Source: CAD feature listing. Evaluate the final solid. Frame: model axes, mm. A direction names the side the tool comes from. Give positions to 0.01 mm unless a question says otherwise; leave off trailing zeros. Loops run counter-clockwise (first coordinate to the right, second up) from the corner with the lowest first, then second, coordinate; pieces in that order, holes last.
```python
from build123d import *

# Parameters (mm, degrees)
F0_W     = 6.35
F0_H     = 34.29
F1_DEPTH = 9.525
F3_DEPTH = 6.351


with BuildPart() as f1:
    # F0 (on Top) → F1 (new body)
    with BuildSketch(Plane.XY):
        Rectangle(F0_W, F0_H)
    extrude(amount=F1_DEPTH)

    # F2 (on face) → F3 (cut, through all)
    with BuildSketch(Plane(origin=(-3.175, 0, 0), x_dir=(0, -1, 0), z_dir=(-1, 0, 0))):
        Polygon((-17.145, 9.525), (-17.145, 6.35), (-10.795, 6.35), (-13.97, 9.525), align=None)
        Polygon((17.145, 9.525), (13.97, 9.525), (10.795, 6.35), (17.145, 6.35), align=None)
    extrude(amount=-F3_DEPTH, mode=Mode.SUBTRACT)


solid = f1.part
```
(1) Section A-A, the plane y = 12. Return the cut outline in (x, z) (3 decimals), then the cut area to 3 significant figures.
A:
outline: (-3.175, 0) - (3.175, 0) - (3.175, 6.35) - (-3.175, 6.35) - close; (-3.175, 7.555) - (3.175, 7.555) - (3.175, 9.525) - (-3.175, 9.525) - close
area: 52.8 mm2
(2) Section C-C, the plane y = -13. Return the cut outline in (x, z) (3 decimals), then the cut area to 3 significant figures.
A:
outline: (-3.175, 0) - (3.175, 0) - (3.175, 6.35) - (-3.175, 6.35) - close; (-3.175, 8.555) - (3.175, 8.555) - (3.175, 9.525) - (-3.175, 9.525) - close
area: 46.5 mm2
(3) Section B-B, the plane x = -2. Return the cut outline in (y, z) (3 decimals).
A:
outline: (-17.145, 0) - (17.145, 0) - (17.145, 6.35) - (10.795, 6.35) - (13.97, 9.525) - (-13.97, 9.525) - (-10.795, 6.35) - (-17.145, 6.35) - close
(4) Reachability of faces 5 (the flat face through (0, -14, 6.35)), 6 (the flat face through (-0.044, 12.36, 7.915)), 7 (the flat face through (0, 0, 9.525)) from +Z, -Z, +X, -X, +Y, -Y: full face, straight path, thin tool, end or side. Return the list, or none.
A:
face 5: +X, -X, -Y
face 6: +X, -X, +Y
face 7: +Z, +X, -X, +Y, -Y
(5) Section D-D, the plane z = 8.5. Return the cut outline in (x, y) (3 decimals), then the cut area to 3 significant figures.
A:
outline: (-3.175, -12.945) - (3.175, -12.945) - (3.175, 12.945) - (-3.175, 12.945) - close
area: 164 mm2
(6) First-contact query: pin 1 (1.9 mm diameter, centred on x = 1.5, y = 15, fed in from +Z). Flat tip, straight axial feed; report the tip coordinate or a pass-through.
A:
pin 1: stops at z = 6.35
(7) Ray query, line 1 along Z through (x, y) = (1.5, -12.5) (3 decimals); line 2 along Z through (x, y) = (-0.5, -11.5) (3 decimals); line 3 along Z through (x, y) = (-2.5, 15). Return the intervals inside material, ascending.
A:
line 1: z = 0 to 6.35, 8.055 to 9.525
line 2: z = 0 to 6.35, 7.055 to 9.525
line 3: z = 0 to 6.35
(8) Mould query, pull axis Z, two halves, no side actions, for faces 1 (the flat face through (-0.044, -12.405, 7.96)), 2 (the flat face through (0, 14, 6.35)), 3 (the flat face through (0, 0, 0)), 4 (the flat face through (3.175, 0, 5)). Classes: pulls with the +Z half, pulls with the -Z half, needs draft (parallel to the pull), parting line crosses it, or undercut.
A:
face 1: undercut
face 2: undercut
face 3: pulls with the -Z half
face 4: needs draft
